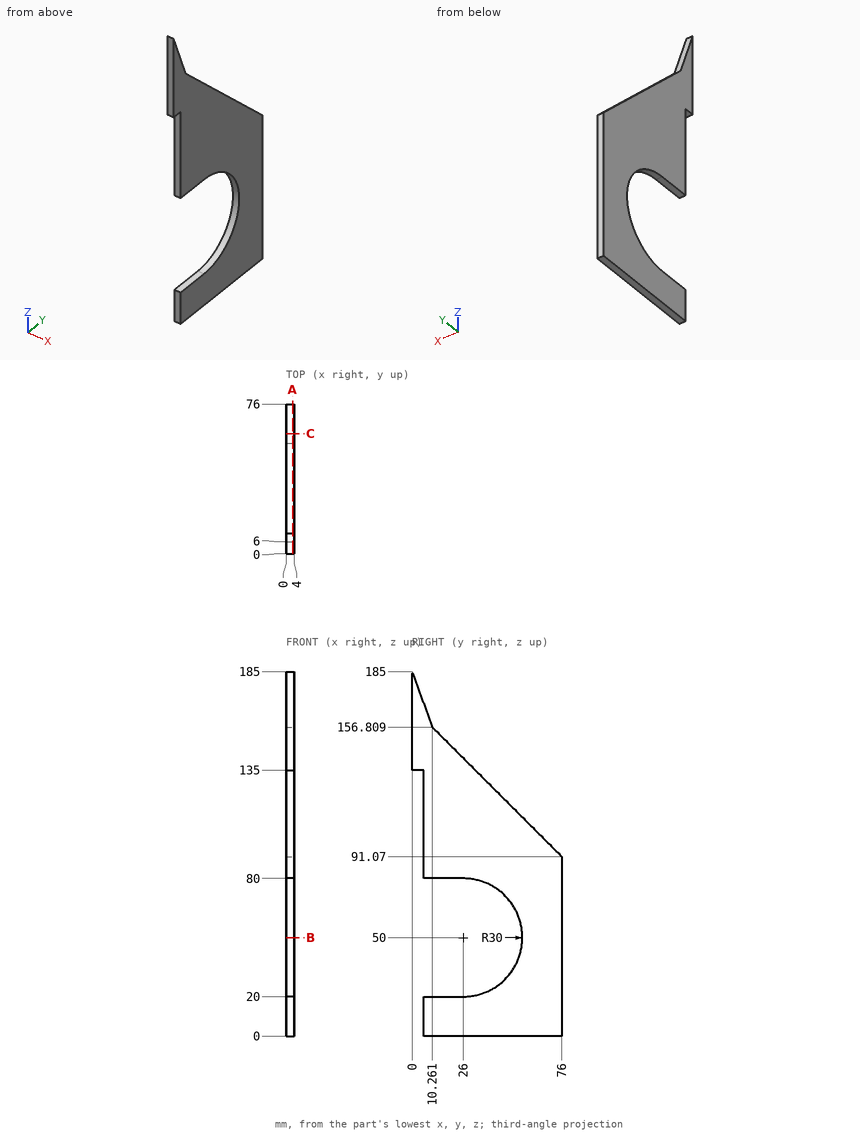
The drawing under review shows one solid part. Ordinate dimensions are in mm from its lowest x, y, z. Coordinates: 2 decimals unless noted, no trailing zeros. Write each loop counter-clockwise with the first axis right and the second up, starting at its lowest first coordinate (ties: lowest second). Pieces come first, ordered by that corner, then holes. Notation, with made-up numbers: (77, -30) - (102, -30) arc R21 cw to (102, -6) - close; hole circle Ø7 at (14.5, -10). An arc over 180 degrees is marked (long way). Answer in a Markdown table with one row per item. Add a question column.
Q1. We need section A-A, the plane x = 3.2. State the section outline as (y, z) points, and give its area (3 significant figures).
Q2. We need section C-C, the plane y = 61. State the section outline as (x, z) points, and give its area (3 significant figures).
Q3. We need section B-B, the plane z = 50. State the section outline as (x, y) points.
Q4. For probe 1 along Z at (x, y) = (2.35, 12); probe 2 along Z at (x, y) = (3.25, 28) (1 decimal); probe 3 along Y at (x, z) = (3.5, 148.5), list the stretches that pass through material, from the lowest coordinate up.
Q5. For P1, Ø1.2, axis at x = 3, z = 112, coming from the -Y side; P2, Ø2, axis at x = 1.5, y = 2, coming from the -Z side; P3, Ø2, axis at x = 0.5, y = 21.5, coming from the +Z side; P4, Ø2, axis at x = 1, y = 13.5, coming from the -Z side, all flat-tipped, find the tip position at first contact; note any pin that passes through.
Answer list:
| question | item | result |
|---|---|---|
| 1 | outline | (0, 135) - (6, 135) - (6, 80) - (26, 80) arc R30 cw to (26, 20) - (6, 20) - (6, 0) - (76, 0) - (76, 91.07) - (10.26, 156.81) - (0, 185) - close |
| 1 | area | 6,480 mm2 |
| 2 | outline | (0, 0) - (4, 0) - (4, 106.07) - (0, 106.07) - close |
| 2 | area | 424 mm2 |
| 3 | outline | (0, 56) - (4, 56) - (4, 76) - (0, 76) - close |
| 4 | probe 1 | z = 0 to 20, 80 to 155.07 |
| 4 | probe 2 | z = 0 to 20.1, 79.9 to 139.1 |
| 4 | probe 3 | y = 0 to 18.57 |
| 5 | P1 | stops at y = 6 |
| 5 | P2 | stops at z = 135 |
| 5 | P3 | stops at z = 146.57 |
| 5 | P4 | stops at z = 0 |
